Check sheet for the drawn part. Datum: minimum x, y, z corner. Units: mm. Round coordinates to 2 decimals unless told otherwise and drop trailing zeros. Write each loop counter-clockwise with the first axis right and the second up, starting at its lowest first coordinate (ties: lowest second). Pieces come first, ordered by that corner, then holes. Notation, with made-up numbers: (25.5, 79.5) - (63.5, 79.5) arc R27 ccw to (63.5, 106.5) - close; hole circle Ø4 at (49.5, 63.25). An arc over 180 degrees is marked (long way). Answer as a JSON object with one key per item and string values.
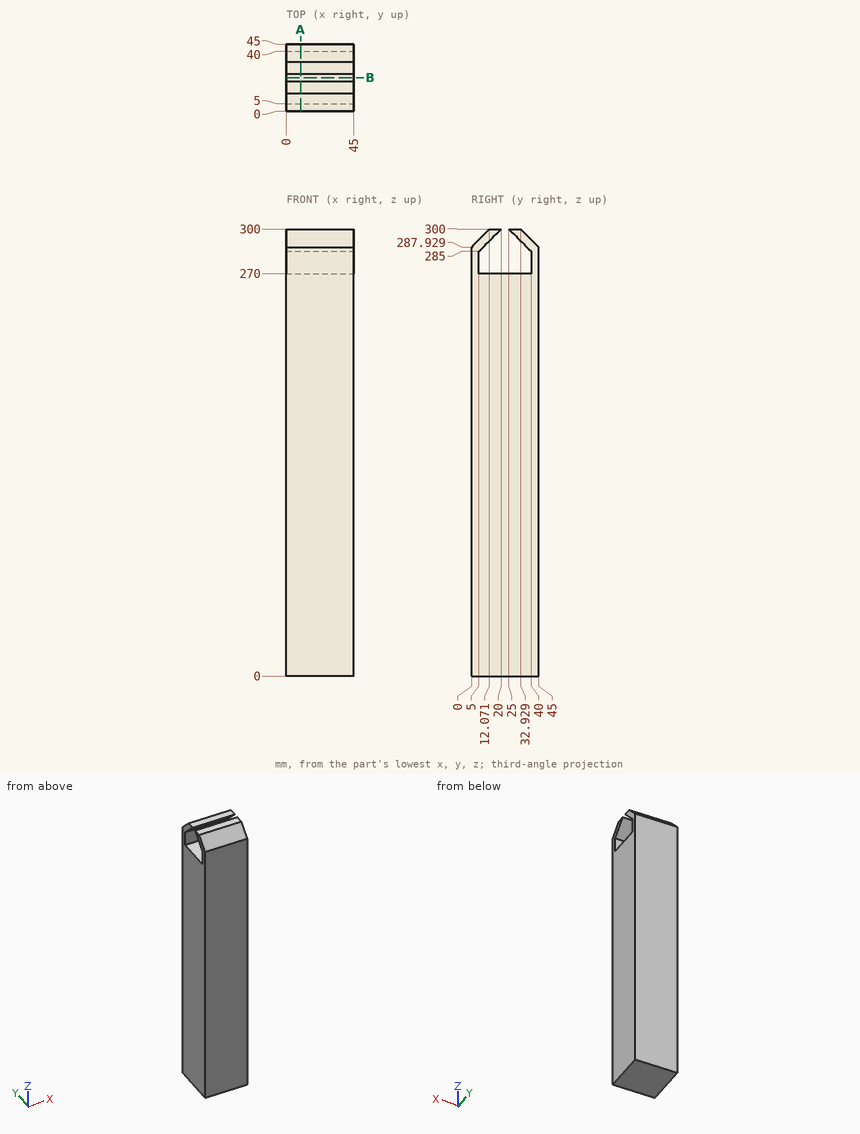
Q1. Material ranges on line 1 along Z through (x, y) = (12, 18.5); line 2 along Z through (x, y) = (15, 8); line 3 along Z through (x, y) = (14, 21), recorded low to high. Write a range as [from, to].
Geometry check:
{"line 1": "z = [0, 270], [298.5, 300]", "line 2": "z = [0, 270], [288, 295.93]", "line 3": "z = [0, 270]"}
Q2. Section check B-B, the plane y = 22.5. Record the cut outline in (x, z), then the cut area to 4 significant figures.
Geometry check:
{"outline": "(0, 0) - (45, 0) - (45, 270) - (0, 270) - close", "area": "12,150 mm2"}
Q3. Section check A-A, the plane x = 9.5. Record the cut outline in (y, z), then the cut area to 3 significant figures.
Geometry check:
{"outline": "(0, 0) - (45, 0) - (45, 287.93) - (32.93, 300) - (25, 300) - (40, 285) - (40, 270) - (5, 270) - (5, 285) - (20, 300) - (12.07, 300) - (0, 287.93) - close", "area": "12,500 mm2"}
